```python
from build123d import *

# Parameters (mm, degrees)
SKETCH2_R                = 38.1
BOSS_EXTRUDE1_DEPTH      = 31.75
SKETCH5_R                = 63.5
BOSS_EXTRUDE2_DEPTH      = 6.35
CUT_EXTRUDE1_DEPTH       = 110.985226281
CUT_EXTRUDE1_DEPTH_BACK  = 110.985226281
SKETCH7_R                = 1.5875
CUT_EXTRUDE2_DEPTH       = 114.769602707
SKETCH9_R                = 4.7625
CUT_EXTRUDE3_DEPTH       = 19.05
CHAMFER1_SIZE            = 3.175
CHAMFER1_OF_MIRROR1_SIZE = 3.175


with BuildPart() as part:
    # Sketch2 → Boss-Extrude1 (new, symmetric)
    with BuildSketch(Plane.XY):
        Circle(SKETCH2_R)
    extrude(amount=BOSS_EXTRUDE1_DEPTH, both=True)

    # Sketch5 → Boss-Extrude2 (add)
    with BuildSketch(Plane.XY.offset(31.75)):
        Circle(SKETCH5_R)
    extrude(amount=BOSS_EXTRUDE2_DEPTH)

    # Sketch7 → Cut-Extrude1 (cut, two sides: drawn at the far end of the back side and taken through both)
    with BuildSketch(Plane(origin=(0, 0, 31.75), x_dir=(-1, 0, 0), z_dir=(0, 0, -1)).offset(-CUT_EXTRUDE1_DEPTH_BACK)):
        with Locations((0, 38.1)):
            Circle(SKETCH7_R)
    extrude(amount=CUT_EXTRUDE1_DEPTH + CUT_EXTRUDE1_DEPTH_BACK, mode=Mode.SUBTRACT)

    # Sketch8 → Cut-Extrude2 (cut, through all)
    with BuildSketch(Plane(origin=(0, 0, -31.75), x_dir=(-1, 0, 0), z_dir=(0, 0, -1))):
        with BuildLine():
            Line((-1.322875656, 1.5), (1.322875656, 1.5))
            ThreePointArc((1.322875656, 1.5), (0, -2), (-1.322875656, 1.5))
        make_face()
    extrude(amount=-CUT_EXTRUDE2_DEPTH, mode=Mode.SUBTRACT)

    # Sketch9 → Cut-Extrude3 (cut)
    with BuildSketch(Plane(origin=(0, 0, -31.75), x_dir=(-1, 0, 0), z_dir=(0, 0, -1))):
        with Locations((0, 19.05)):
            Circle(SKETCH9_R)
    cut_extrude3 = extrude(amount=-CUT_EXTRUDE3_DEPTH, mode=Mode.SUBTRACT)

    # Chamfer1
    chamfer1_edges = [part.edges().sort_by_distance(p)[0] for p in [
        (4.7625, 19.05, -31.75),
    ]]
    chamfer(chamfer1_edges, length=CHAMFER1_SIZE)

    # Mirror1: Cut-Extrude3 across plane
    add(cut_extrude3.mirror(Plane.ZX), mode=Mode.SUBTRACT)

    # Chamfer1 of Mirror1
    chamfer1_of_mirror1_edges = [part.edges().sort_by_distance(p)[0] for p in [
        (4.7625, -19.05, -31.75),
    ]]
    chamfer(chamfer1_of_mirror1_edges, length=CHAMFER1_OF_MIRROR1_SIZE)


solid = part.part
```
Part model, mm, in its own coordinate system. A direction names the side the tool comes from. Round coordinates to 2 decimals unless told otherwise and drop trailing zeros. Loops run counter-clockwise (first coordinate to the right, second up) from the corner with the lowest first, then second, coordinate; pieces in that order, holes last.
Item 1: Drop flat-ended pins along their axis: P1, Ø8, axis at y = 0, z = -21.5, coming from the +X side; P2, Ø11, axis at x = 0, y = 19.05, coming from the -Z side; P3, Ø1.5, axis at x = 22.5, z = -6, coming from the -Y side; P4, Ø4.5, axis at x = 0, y = 0, coming from the -Z side. Give the stop position or say it passes through.
Item 2: Cut at A-A, the plane z = -20. State how many separate pieces and enclosed holes the cut face has, then the cut area to 3 significant figures.
Item 3: Cut at D-D, the plane x = 50.5. Give the cut face in (y, z).
Item 4: Mould opens along X. For faces 1 (the face through (-13.77, -61.99, 34.88)), 2 (the face through (13, 1, 38.1)), 3 (the face through (0.6, -23.9, -28.7)) say: +X half, -X half, draft (parallel to the pull), parting line (faces both ways), or undercut.
Item 5: 3-axis set-ups, long thin cutter, end or side, ignore diameter. For faces 4 (the face through (8, 1, -31.75)), 5 (the face through (0, -19, -12.7)): which of +Z, -Z, +X, -X, +Y, -Y reach the whole face in a straight line?
Item 6: Drill centre lines: line 1 (Y direction, x = 0, z = -20); line 2 (Y direction, x = 0, z = -2); line 3 (Z direction, x = -39, y = -4.5). Where is each one in solid material? Low to high.
Item 7: Cut at C-C, the plane z = 28.5. Give the cut face in (x, y) (1 decimal), then the cut area to 3 significant figures.
A:
1. P1: stops at x = 38.1
1. P2: stops at z = -29.31
1. P3: stops at y = -31.28
1. P4: stops at z = -31.75
2. separate pieces: 1
2. enclosed holes: 3
2. area: 4,400 mm2
3. outline: (-38.5, 31.75) - (38.5, 31.75) - (38.5, 38.1) - (-38.5, 38.1) - close
4. face 1: parting line
4. face 2: draft
4. face 3: undercut
5. face 4: -Z, +X, -X, +Y, -Y
5. face 5: -Z
6. line 1: y = -38.1 to -23.81, -14.29 to -2, 1.5 to 14.29, 23.81 to 36.51
6. line 2: y = -38.1 to -2, 1.5 to 36.51
6. line 3: z = 31.75 to 38.1
7. outline: (-1.6, 38.1) arc R38.1 ccw (long way) to (1.6, 38.1) arc R1.6 cw to start; hole (-1.3, 1.5) arc R2 ccw (long way) to (1.3, 1.5) - close
7. area: 4,540 mm2
